Autodesk Inventor part; units mm, degrees
ref_plane "YZ Plane" through (0, 0, 0) normal (1, 0, 0) x (0, 1, 0)
ref_plane "XZ Plane" through (0, 0, 0) normal (0, 1, 0) x (-1, 0, 0)
ref_plane "XY Plane" through (0, 0, 0) normal (0, 0, 1) x (1, 0, 0)
sketch "Sketch2" plane through (0, 0, 0) normal (0, 0, 1) x (1, 0, 0)
  circle A0 centre (0, 0) radius 60
  circle A1 centre (0, 0) radius 97.5
  dimension "d25" = 120
  dimension "d27" = 195
extrude "Plate2" add sketch "Sketch2" along normal blind 6
sketch "Sketch3" plane through (0, 0, 6) normal (0, 0, 1) x (1, 0, 0)
  circle A0 centre (-80, 0) radius 8.5
  circle A1 centre (0, 0) radius 80 construction
  dimension "d28" = 160
  dimension "d15" = 17
extrude "Cut1" cut sketch "Sketch3" against normal blind 6
pattern_circular "Circular Pattern1" count 4 over 360 about axis through (0, 0, -10) along (0, 0, 1) of "Cut1"
equation "\"d17\" = Thickness"
equation "\"d14\" = Thickness"
equation "\"BendReliefWidth\" = Thickness"
equation "\"BendReliefDepth\" = 0.5 * Thickness"
equation "\"CornerReliefSize\" = 4 * Thickness"
equation "\"MinimumRemnant\" = 2 * Thickness"
equation "\"TransitionRadius\" = BendRadius"
equation "\"JacobiRadiusSize\" = BendRadius"
equation "\"GapSize\" = Thickness"
properties part number "PRS 9431 FDS flange DN90_D1200" material "Steel"
Design review of the part built by this model. Coordinates are the model's own, in mm. Give positions to 0.01 mm unless a question says otherwise; leave off trailing zeros. Write each loop counter-clockwise with the first axis right and the second up, starting at its lowest first coordinate (ties: lowest second). Pieces come first, ordered by that corner, then holes. Notation, with made-up numbers: M 82.5,-1.75 L 105.5,-1.75 A22 ccw 105.5,20.25 Z; hole C 54.5,13.5 d6. An arc over 180 degrees is marked long. Answer as a JSON object with one key per item and string values. Group by question number.
1) Clearance check with flat-ended pins moving along their axes: pin 1 Ø22 at (x, y) = (-80, 0) entering from -Z; pin 2 Ø1.5 at (x, z) = (39.5, 4.5) entering from +Y; pin 3 Ø2 at (x, z) = (-59, 3) entering from -Y; pin 4 Ø13.5 at (x, y) = (0, 80) entering from +Z. State where each tip first meets the part, or that it passes through.
2) We need section A-A (x = 0). Give the boundary of the cut face in (y, z), and give its area (3 significant figures).
3) We need section D-D (z = 1.8). Give the boundary of the cut face in (x, y), and give its area (3 significant figures).
4) Mouldability with a two-part tool opening along Y and no side actions: class faces 1 (the face through (0.37, 88.49, 3.04)), 2 (the face through (-77.37, 59.33, 2.96)), 3 (the face through (-45, -42, 6)) as released by +Y, released by -Y, zero draft, split by the parting line, or undercut.
5) For line 1 along X through (y, z) = (5.5, 2.25); line 2 along X through (y, z) = (15, 4.4); line 3 along X through (y, z) = (-21, 1.6), list the stretches that pass through material, from the lowest coordinate up.
6) We need section B-B (y = -43.5). Give the boundary of the cut face in (x, z).
7) We need section C-C (x = 30). Give the boundary of the cut face in (y, z).
Answer key:
{
 "1": {"pin 1": "stops at z = 0", "pin 2": "stops at y = 89.47", "pin 3": "stops at y = -78.37", "pin 4": "passes through"},
 "2": {"outline": "M -97.5,0 L -88.5,0 L -88.5,6 L -97.5,6 Z; M -71.5,0 L -60,0 L -60,6 L -71.5,6 Z; M 60,0 L 71.5,0 L 71.5,6 L 60,6 Z; M 88.5,0 L 97.5,0 L 97.5,6 L 88.5,6 Z", "area": "246 mm²"},
 "3": {"outline": "C 0,0 d195; hole C -80,0 d17; hole C 0,0 d120; hole C 0,-80 d17; hole C 0,80 d17; hole C 80,0 d17", "area": "17,600 mm²"},
 "4": {"face 1": "undercut", "face 2": "split by the parting line", "face 3": "zero draft"},
 "5": {"line 1": "x = -97.34 to -86.48, -73.52 to -59.75, 59.75 to 73.52, 86.48 to 97.34", "line 2": "x = -96.34 to -58.09, 58.09 to 96.34", "line 3": "x = -95.21 to -56.2, 56.2 to 95.21"},
 "6": {"outline": "M -87.26,0 L -41.32,0 L -41.32,6 L -87.26,6 Z; M 41.32,0 L 87.26,0 L 87.26,6 L 41.32,6 Z"},
 "7": {"outline": "M -92.77,0 L -51.96,0 L -51.96,6 L -92.77,6 Z; M 51.96,0 L 92.77,0 L 92.77,6 L 51.96,6 Z"}
}
